Read the model definition and answer for the solid it produces. Units are mm, in the model's axes. Face numbers are marked on the shaded views. A direction names the side the tool comes from. Round coordinates to 2 decimals unless told otherwise and drop trailing zeros. Write each loop counter-clockwise with the first axis right and the second up, starting at its lowest first coordinate (ties: lowest second). Pieces come first, ordered by that corner, then holes. Notation, with made-up numbers: (42.5, 26) -> (56.5, 26) arc R25 ccw to (56.5, 57) -> close; hole circle Ø1 at (73.25, -15.5). An arc over 180 degrees is marked (long way). Return JSON: item names as keys, results as strings. Group by question number.
(1) Given pin 1 (1.5 mm diameter, centred on y = -10, z = 4, fed in from +X); pin 2 (5 mm diameter, centred on x = -26.63, y = -8.65, fed in from +Z); pin 3 (1 mm diameter, centred on x = -4.5, z = 3, fed in from -Y); pin 4 (1 mm diameter, centred on x = 0, z = 3.5, fed in from -Y), each flat-ended and moving along its own axis, determine where each tip first touches the part or whether it passes through.
(2) A cutting plane is placed at A-A on y = 0. Give the vertices of the cut face in (x, z) (3 decimals), then the cut area to 3 significant figures.
(3) For the marked faces 1 and 2, determine the directions among +Z, -Z, +X, -X, +Y, -Y from which every point of the face is accessible in a straight line to the end or side of a thin tool.
(4) A cutting plane is placed at B-B on x = 0. Give the vertices of the cut face in (y, z) (3 decimals).
(5) A cutting plane is placed at D-D on z = 3.9. Give the vertices of the cut face in (x, y) (3 decimals), then the cut area to 3 significant figures.
(6) A cutting plane is placed at C-C on x = -17.5. Give the vertices of the cut face in (y, z).
(7) Straight lines are drawn through the part: line 1 (Y direction, x = 0, z = 4.8) (3 decimals); line 2 (Y direction, x = 0, z = 0.7); line 3 (X direction, y = -27, z = 4.1). For each, find the intervals that lie inside material, in ascending order.
```python
from build123d import *

# Parameters (mm, degrees)
SKETCH_1_R      = 34.5
SKETCH_1_R_2    = 13
SKETCH_1_R_3    = 2
EXTRUDE_1_DEPTH = 2
SKETCH_2_R      = 32.5
SKETCH_2_R_2    = 13.625
SKETCH_2_R_3    = 2
EXTRUDE_2_DEPTH = 4


with BuildPart() as part:
    # 草图1 → 凸台-拉伸1 (new body)
    with BuildSketch(Plane.XY):
        Circle(SKETCH_1_R)
        Circle(SKETCH_1_R_2, mode=Mode.SUBTRACT)
        with Locations((0, -28)):
            Circle(SKETCH_1_R_3, mode=Mode.SUBTRACT)
        with Locations((-26.629582456, -8.652475842)):
            Circle(SKETCH_1_R_3, mode=Mode.SUBTRACT)
        with Locations((-16.457987064, 22.652475842)):
            Circle(SKETCH_1_R_3, mode=Mode.SUBTRACT)
        with Locations((16.457987064, 22.652475842)):
            Circle(SKETCH_1_R_3, mode=Mode.SUBTRACT)
        with Locations((26.629582456, -8.652475842)):
            Circle(SKETCH_1_R_3, mode=Mode.SUBTRACT)
    extrude(amount=EXTRUDE_1_DEPTH)

    # 草图2 → 凸台-拉伸2 (add)
    with BuildSketch(Plane.XY.offset(2)):
        Circle(SKETCH_2_R)
        Circle(SKETCH_2_R_2, mode=Mode.SUBTRACT)
        with Locations((0, -28)):
            Circle(SKETCH_2_R_3, mode=Mode.SUBTRACT)
        with Locations((-26.629582456, -8.652475842)):
            Circle(SKETCH_2_R_3, mode=Mode.SUBTRACT)
        with Locations((-16.457987064, 22.652475842)):
            Circle(SKETCH_2_R_3, mode=Mode.SUBTRACT)
        with Locations((16.457987064, 22.652475842)):
            Circle(SKETCH_2_R_3, mode=Mode.SUBTRACT)
        with Locations((26.629582456, -8.652475842)):
            Circle(SKETCH_2_R_3, mode=Mode.SUBTRACT)
    extrude(amount=EXTRUDE_2_DEPTH)


solid = part.part
```
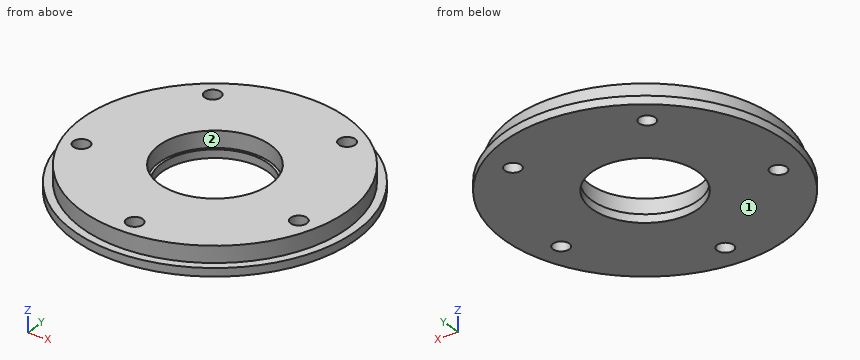
Checks:
{
 "1": {"pin 1": "stops at x = 31.16", "pin 2": "stops at z = 6", "pin 3": "stops at y = -32.25", "pin 4": "stops at y = -32.5"},
 "2": {"outline": "(-34.5, 0) -> (-13, 0) -> (-13, 2) -> (-13.625, 2) -> (-13.625, 6) -> (-32.5, 6) -> (-32.5, 2) -> (-34.5, 2) -> close; (13, 0) -> (34.5, 0) -> (34.5, 2) -> (32.5, 2) -> (32.5, 6) -> (13.625, 6) -> (13.625, 2) -> (13, 2) -> close", "area": "237 mm^2"},
 "3": {"face 1": "-Z, +X, -X, +Y, -Y", "face 2": "+Z"},
 "4": {"outline": "(-34.5, 0) -> (-30, 0) -> (-30, 6) -> (-32.5, 6) -> (-32.5, 2) -> (-34.5, 2) -> close; (-26, 0) -> (-13, 0) -> (-13, 2) -> (-13.625, 2) -> (-13.625, 6) -> (-26, 6) -> close; (13, 0) -> (34.5, 0) -> (34.5, 2) -> (32.5, 2) -> (32.5, 6) -> (13.625, 6) -> (13.625, 2) -> (13, 2) -> close"},
 "5": {"outline": "circle Ø65 at (0, 0); hole circle Ø4 at (-26.63, -8.652); hole circle Ø4 at (-16.458, 22.652); hole circle Ø27.25 at (0, 0); hole circle Ø4 at (0, -28); hole circle Ø4 at (16.458, 22.652); hole circle Ø4 at (26.63, -8.652)", "area": "2,670 mm^2"},
 "6": {"outline": "(-29.73, 0) -> (20.95, 0) -> (20.95, 6) -> (-27.39, 6) -> (-27.39, 2) -> (-29.73, 2) -> close; (24.36, 0) -> (29.73, 0) -> (29.73, 2) -> (27.39, 2) -> (27.39, 6) -> (24.36, 6) -> close"},
 "7": {"line 1": "y = -32.5 to -30, -26 to -13.625, 13.625 to 32.5", "line 2": "y = -34.5 to -30, -26 to -13, 13 to 34.5", "line 3": "x = -18.09 to -1.73, 1.73 to 18.09"}
}
